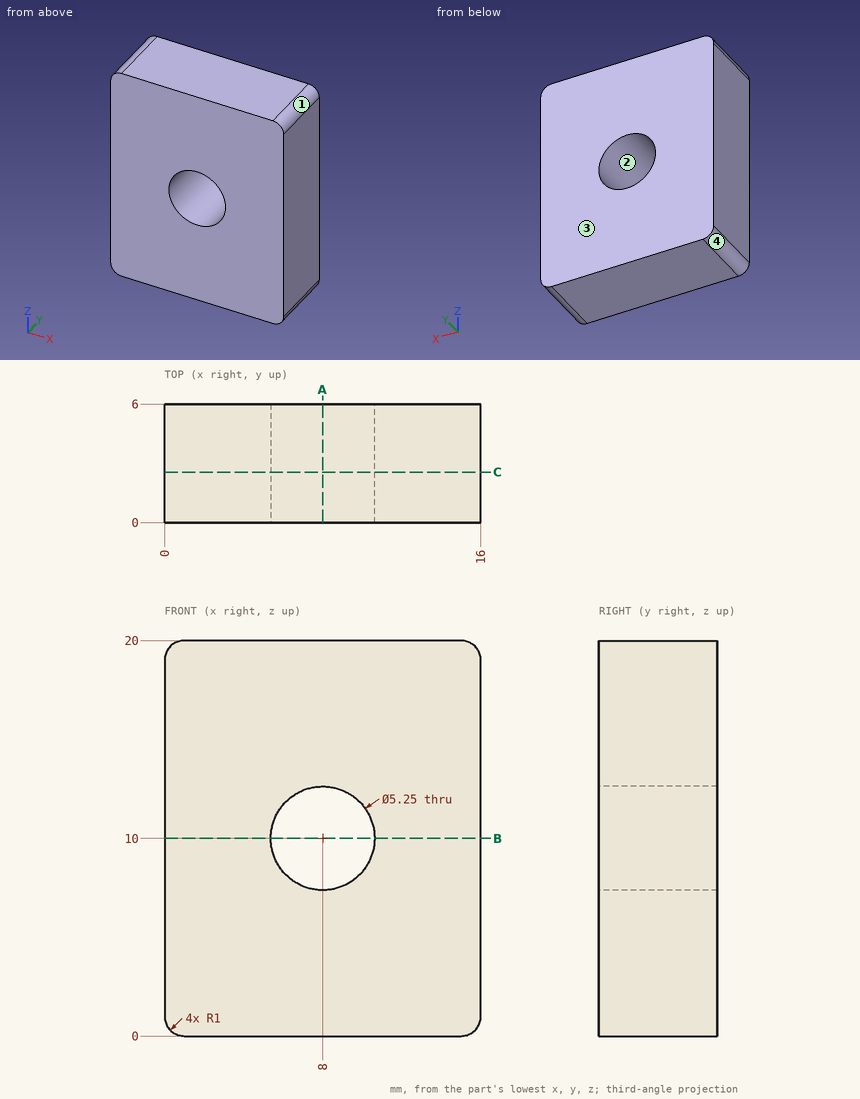
Check sheet for the drawn part. Datum: minimum x, y, z corner. Units: mm. Coordinates: 2 decimals unless noted, no trailing zeros. Loops run counter-clockwise (first coordinate to the right, second up) from the corner with the lowest first, then second, coordinate; pieces in that order, holes last. Notation, with made-up numbers: (56, 8.5) -> (89, 8.5) arc R18 ccw to (89, 25.5) -> close; hole circle Ø3 at (81, 19.5). An arc over 180 degrees is marked (long way). Answer as a JSON object with one key per item and string values. Group by question number.
Item 1: Depth check by flat-ended pin: pin 1 (2 mm diameter, centred on x = 2, y = 3, fed in from -Z). Enter the tip coordinate at first touch or a pass-through.
Item 2: Scan lines: probe 1 along Z at (x, y) = (8, 4) (3 decimals); probe 2 along X at (y, z) = (3.2, 10) (3 decimals); probe 3 along X at (y, z) = (3.15, 19.25). Record each from-to range of solid material in increasing order.
Item 3: Mould release check, pull along X, two halves, no side actions. Record for the marked faces 1, 2, 3 and 4: +X half, -X half, draft (parallel to the pull), parting line (faces both ways), or undercut.
Item 4: Sectioned sample at B-B on z = 10. Record the boundary of the cut face in (x, y) (3 decimals).
Item 5: Sectioned sample at C-C on y = 2.55. Record the boundary of the cut face in (x, z) (3 decimals), plus the area to 3 significant figures.
Item 6: Sectioned sample at A-A on x = 8. Record the boundary of the cut face in (y, z) (3 decimals).
Evaluation:
{
 "1": {"pin 1": "stops at z = 0"},
 "2": {"probe 1": "z = 0 to 7.375, 12.625 to 20", "probe 2": "x = 0 to 5.375, 10.625 to 16", "probe 3": "x = 0.03 to 15.97"},
 "3": {"face 1": "+X half", "face 2": "undercut", "face 3": "draft", "face 4": "-X half"},
 "4": {"outline": "(0, 0) -> (5.375, 0) -> (5.375, 6) -> (0, 6) -> close; (10.625, 0) -> (16, 0) -> (16, 6) -> (10.625, 6) -> close"},
 "5": {"outline": "(0, 1) arc R1 ccw to (1, 0) -> (15, 0) arc R1 ccw to (16, 1) -> (16, 19) arc R1 ccw to (15, 20) -> (1, 20) arc R1 ccw to (0, 19) -> close; hole circle Ø5.25 at (8, 10)", "area": "297 mm²"},
 "6": {"outline": "(0, 0) -> (6, 0) -> (6, 7.375) -> (0, 7.375) -> close; (0, 12.625) -> (6, 12.625) -> (6, 20) -> (0, 20) -> close"}
}
